CAD build for the part. Positions are in the model's coordinates, mm. Face numbers are marked on the shaded views. A direction names the side the tool comes from. Coordinates: 2 decimals unless noted, no trailing zeros. Loops run counter-clockwise (first coordinate to the right, second up) from the corner with the lowest first, then second, coordinate; pieces in that order, holes last.
1) Saw through at A-A, the plane z = -12.5. Write the cut outline in (x, y), and give its area (3 significant figures).
2) Wall check: line 1 along Z through (x, y) = (2.65, 0); line 2 along X through (y, z) = (-0.25, -9); line 3 along Z through (x, y) = (-2.5, 2.75). Give the ranges that are in metal, low to high.
3) Pin check, flat tips, straight feed: pin 1 Ø3 at (x, y) = (-3, -2.5) entering from -Z; pin 2 Ø3 at (y, z) = (2, 0) entering from -X; pin 3 Ø4 at (x, z) = (-4, 1.5) entering from -Y. Stop position of each tip, or through.
4) Saw through at C-C, the plane x = 0. Write the cut outline in (y, z).
5) Saw through at B-B, the plane y = 0. Write the cut outline in (x, z).
6) Which spindle directions (+Z, -Z, +X, -X, +Y, -Y) get a long thin tool onto all of the face, cutting with end or side? Do the marked faces 4, 5 and 6. Say none if no direction does.
7) Saw through at D-D, the plane x = 2.5. Write the cut outline in (y, z).
8) Two-plate mould, pull along X, no slides. Class the marked faces 1, 2 and 3: +X half, -X half, draft (parallel to the pull), parting line (faces both ways), or undercut.
```python
from build123d import *

# Parameters (mm, degrees)
SKETCH1_R           = 6.1
BOSS_EXTRUDE1_DEPTH = 10.5
SKETCH2_W           = 15.5
SKETCH2_H           = 15.5
BOSS_EXTRUDE2_DEPTH = 4
CUT_EXTRUDE1_DEPTH  = 4
SKETCH4_R           = 0.8
CUT_EXTRUDE2_DEPTH  = 5.5


with BuildPart() as part:
    # Sketch1 → Boss-Extrude1 (new, symmetric)
    with BuildSketch(Plane.XY):
        with Locations(Location((0, 0, 0), (0, 0, 180))):
            Circle(SKETCH1_R)
    extrude(amount=BOSS_EXTRUDE1_DEPTH, both=True)

    # Sketch2 → Boss-Extrude2 (add)
    with BuildSketch(Plane(origin=(0, 0, -10.5), x_dir=(-1, 0, 0), z_dir=(0, 0, -1))):
        Rectangle(SKETCH2_W, SKETCH2_H)
    extrude(amount=BOSS_EXTRUDE2_DEPTH)

    # Sketch3 → Cut-Extrude1 (cut)
    with BuildSketch(Plane(origin=(0, 0, -14.5), x_dir=(-1, 0, 0), z_dir=(0, 0, -1))):
        with BuildLine():
            Line((-0.75, 5), (1.25, 5))
            ThreePointArc((1.25, 5), (4.078427125, 3.828427125), (5.25, 1))
            Line((5.25, 1), (5.25, -1))
            ThreePointArc((5.25, -1), (4.078427125, -3.828427125), (1.25, -5))
            Line((1.25, -5), (-0.75, -5))
            Line((-0.75, -5), (-0.75, 5))
        make_face()
    extrude(amount=-CUT_EXTRUDE1_DEPTH, mode=Mode.SUBTRACT)

    # Sketch4 → Cut-Extrude2 (cut)
    with BuildSketch(Plane.ZY.offset(-0.75)):
        with Locations(Location((-12.5, 0, 0), (0, 0, 270))):
            Circle(SKETCH4_R)
    extrude(amount=-CUT_EXTRUDE2_DEPTH, mode=Mode.SUBTRACT)


solid = part.part
```
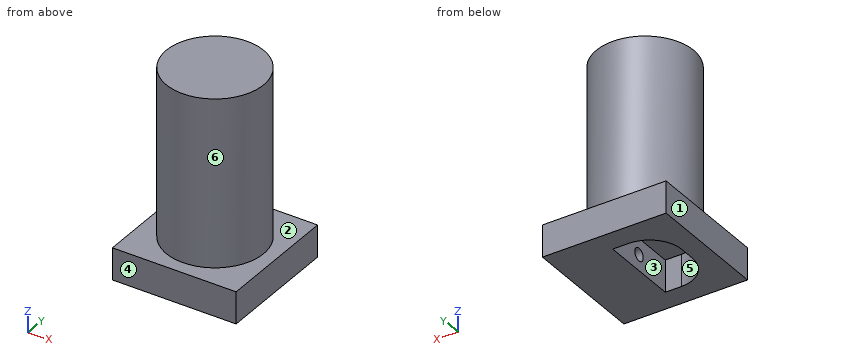
Data:
1. outline: (-7.75, -7.75) - (7.75, -7.75) - (7.75, 7.75) - (-7.75, 7.75) - close; hole (-5.25, -1) arc R4 ccw to (-1.25, -5) - (0.75, -5) - (0.75, -0.8) - (6.25, -0.8) - (6.25, 0.8) - (0.75, 0.8) - (0.75, 5) - (-1.25, 5) arc R4 ccw to (-5.25, 1) - close
1. area: 178 mm2
2. line 1: z = -14.5 to -13.3, -11.7 to 10.5
2. line 2: x = -6.09 to 6.09
2. line 3: z = -10.5 to 10.5
3. pin 1: stops at z = -10.5
3. pin 2: stops at x = -6.08
3. pin 3: stops at y = -5.76
4. outline: (-7.75, -14.5) - (-5, -14.5) - (-5, -10.5) - (5, -10.5) - (5, -14.5) - (7.75, -14.5) - (7.75, -10.5) - (6.1, -10.5) - (6.1, 10.5) - (-6.1, 10.5) - (-6.1, -10.5) - (-7.75, -10.5) - close
5. outline: (-7.75, -14.5) - (-5.25, -14.5) - (-5.25, -10.5) - (0.75, -10.5) - (0.75, -11.7) - (6.25, -11.7) - (6.25, -13.3) - (0.75, -13.3) - (0.75, -14.5) - (7.75, -14.5) - (7.75, -10.5) - (6.1, -10.5) - (6.1, 10.5) - (-6.1, 10.5) - (-6.1, -10.5) - (-7.75, -10.5) - close
6. face 4: +Z, -Z, +X, -X, -Y
6. face 5: -Z
6. face 6: +Z
7. outline: (-7.75, -14.5) - (7.75, -14.5) - (7.75, -10.5) - (5.56, -10.5) - (5.56, 10.5) - (-5.56, 10.5) - (-5.56, -10.5) - (-7.75, -10.5) - close; hole circle Ø1.6 at (0, -12.5)
8. face 1: -X half
8. face 2: draft
8. face 3: undercut
